Could you check a few things on this drawing? It's one solid part, dimensions in mm from its lowest x, y, z. A direction names the side the tool comes from. Give positions to 0.01 mm unless a question says otherwise; leave off trailing zeros. Order: outer loops, then holes, each group sorted by start corner. A loop starts at its lowest first (then second) coordinate and runs counter-clockwise, first axis right, second up. Notation, with made-up numbers: (-4.5, -1.5) -> (40.5, -1.5) arc R26 ccw to (40.5, 15.5) -> close; hole circle Ø9 at (88.25, 7.5). An arc over 180 degrees is marked (long way). Answer as a JSON object with one key per item and string values.
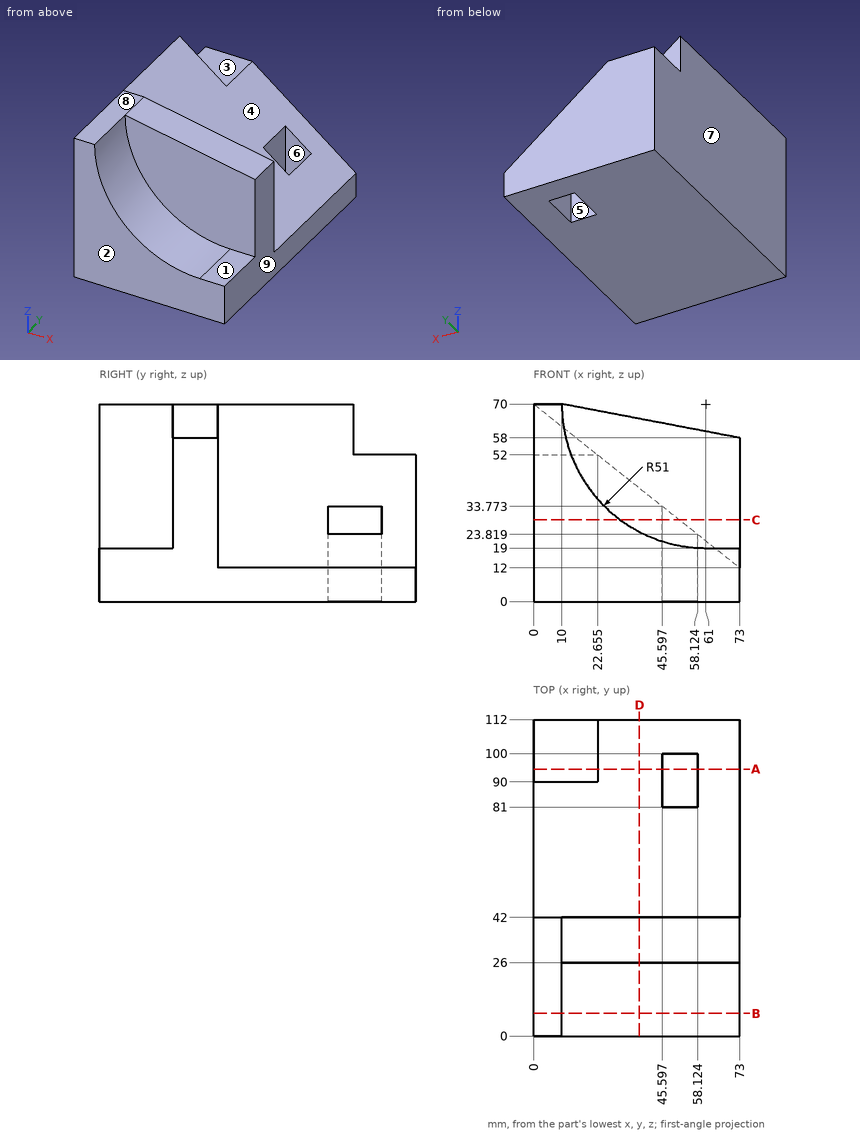
1. Will these pins go through, and if not, where does the flat tip stop? pin 1 Ø6 at (x, y) = (67.5, 11) entering from +Z; pin 2 Ø15.5 at (x, z) = (48, 49.5) entering from -Y; pin 3 Ø21 at (y, z) = (90, 25) entering from +X (1 decimal).
Worked answers:
{"pin 1": "z = 19", "pin 2": "y = 26", "pin 3": "x = 69.9"}
2. If we mould it in two halves opening along X, with no side actions, what happens to the marked faces 6, 7, 8 and 9? For each: +X half, -X half, draft (parallel to the pull), parting line (faces both ways), or undercut.
Worked answers:
{"face 6": "undercut", "face 7": "-X half", "face 8": "draft", "face 9": "+X half"}
3. If we section it at A-A on y = 94.5: Please give me the cut outline in (x, z) (1 decimal), then the cut area to 3 significant figures.
Worked answers:
{"outline": "(0, 0) -> (45.6, 0) -> (45.6, 33.8) -> (22.7, 52) -> (0, 52) -> close; (58.1, 0) -> (73, 0) -> (73, 12) -> (58.1, 23.8) -> close", "area": "2,430 mm²"}
4. Please list where these lines run through material, in increasing order: L1, parallel to Y at x = 64, z = 31.5; L2, parallel to X at y = 22.5, z = 37.5 (1 decimal); L3, parallel to Z at x = 46.5, y = 54 (1 decimal).
Worked answers:
{"L1": "26 to 42", "L2": "0 to 21.7", "L3": "0 to 33.1"}
5. If we section it at C-C on z = 29: Please give me the cut outline in (x, y).
Worked answers:
{"outline": "(0, 0) -> (30.67, 0) -> (30.67, 26) -> (73, 26) -> (73, 42) -> (51.6, 42) -> (51.6, 81) -> (45.6, 81) -> (45.6, 100) -> (51.6, 100) -> (51.6, 112) -> (0, 112) -> close"}
6. For the marked faces 1, 2, 3, 4 and 5, which set-ups out of +Z, -Z, +X, -X, +Y, -Y let a thin tool reach every point of the face, with its end or its side?
Worked answers:
{"face 1": "+Z, +X, -Y", "face 2": "+Z, -Z, +X, -X, -Y", "face 3": "+Z, +X, -X, +Y", "face 4": "+Z, +X, +Y", "face 5": "+Z, -Z"}
7. If we section it at B-B on y = 8: Please give me the cut outline in (x, z).
Worked answers:
{"outline": "(0, 0) -> (73, 0) -> (73, 19) -> (61, 19) arc R51 cw to (10, 70) -> (0, 70) -> close"}
8. If we section it at D-D on x = 37.5: Please give me the cut outline in (y, z) (1 decimal), then the cut area to 3 significant figures.
Worked answers:
{"outline": "(0, 0) -> (112, 0) -> (112, 40.2) -> (42, 40.2) -> (42, 64.8) -> (26, 64.8) -> (26, 24.7) -> (0, 24.7) -> close", "area": "4,490 mm²"}
